from build123d import *

# Parameters (mm, degrees)
SKETCH1_R               = 8.75
SKETCH1_R_2             = 1.5
BOSS_EXTRUDE1_DEPTH     = 8.5
CUT_EXTRUDE2_DEPTH      = 3.5
CUT_EXTRUDE2_DEPTH_BACK = 3.5
CUT_EXTRUDE2_START      = -4.25
SKETCH2_R               = 9
SKETCH2_R_2             = 6
CUT_EXTRUDE5_START      = -0.75
CUT_EXTRUDE5_DEPTH      = 7
CHAMFER1_SIZE           = 0.5


with BuildPart() as part:
    # Sketch1 → Boss-Extrude1 (new body)
    with BuildSketch(Plane(origin=(0, 0, 0), x_dir=(1, 0, 0), z_dir=(0, 1, 0))):
        with Locations(Location((0, 0, 0), (0, 0, 270))):
            Circle(SKETCH1_R)
        with Locations(Location((0, 0, 0), (0, 0, 270))):
            Circle(SKETCH1_R_2, mode=Mode.SUBTRACT)
    extrude(amount=BOSS_EXTRUDE1_DEPTH)

    # Sketch2 → Cut-Extrude2 (cut, two sides: drawn at the far end of the back side and taken through both)
    with BuildSketch(Plane(origin=(0, 8.5, 0), x_dir=(1, 0, 0), z_dir=(0, 1, 0)).offset(CUT_EXTRUDE2_START - CUT_EXTRUDE2_DEPTH_BACK)):
        Circle(SKETCH2_R)
        with Locations(Location((0, 0, 0), (0, 0, 270))):
            Circle(SKETCH2_R_2, mode=Mode.SUBTRACT)
    extrude(amount=CUT_EXTRUDE2_DEPTH + CUT_EXTRUDE2_DEPTH_BACK, mode=Mode.SUBTRACT)

    # Sketch4 → Cut-Extrude5 (cut)
    with BuildSketch(Plane(origin=(0, 8.5, 0), x_dir=(1, 0, 0), z_dir=(0, 1, 0)).offset(CUT_EXTRUDE5_START)):
        with BuildLine():
            ThreePointArc((3.526710889, 4.85410242), (3.180827716, 5.087468432), (2.81956216, 5.296231606))
            Line((2.81956216, 5.296231606), (3.230259184, 4.44607034))
            Line((3.230259184, 4.44607034), (4.165722957, 4.318188538))
            ThreePointArc((4.165722957, 4.318188538), (3.855539591, 4.597261626), (3.526710889, 4.85410242))
        make_face()
        with BuildLine():
            ThreePointArc((4.854101297, 3.526712434), (4.597261012, 3.855540323), (4.318188538, 4.165722957))
            Line((4.318188538, 4.165722957), (4.44607034, 3.230259184))
            Line((4.44607034, 3.230259184), (5.296231606, 2.81956216))
            ThreePointArc((5.296231606, 2.81956216), (5.087467925, 3.180828525), (4.854101297, 3.526712434))
        make_face()
        with BuildLine():
            ThreePointArc((1.85410212, 5.706339048), (1.453033176, 5.821399711), (1.044937393, 5.908308205))
            Line((1.044937393, 5.908308205), (1.698247753, 5.226669153))
            Line((1.698247753, 5.226669153), (2.62744432, 5.394120535))
            ThreePointArc((2.62744432, 5.394120535), (2.246204515, 5.563682708), (1.85410212, 5.706339048))
        make_face()
        with BuildLine():
            ThreePointArc((0.831973127, 5.942038431), (0.416994825, 5.98549207), (-5.4e-08, 6))
            ThreePointArc((-5.4e-08, 6), (-0.416994879, 5.985492066), (-0.831973127, 5.942038431))
            Line((-0.831973127, 5.942038431), (0, 5.495645173))
            Line((0, 5.495645173), (0.831973127, 5.942038431))
        make_face()
        with BuildLine():
            Line((-1.698247753, 5.226669153), (-1.044937393, 5.908308205))
            ThreePointArc((-1.044937393, 5.908308205), (-1.453033133, 5.821399721), (-1.854102038, 5.706339075))
            ThreePointArc((-1.854102038, 5.706339075), (-2.246204475, 5.563682724), (-2.62744432, 5.394120535))
            Line((-2.62744432, 5.394120535), (-1.698247753, 5.226669153))
        make_face()
        with BuildLine():
            Line((-3.230259184, 4.44607034), (-2.81956216, 5.296231606))
            ThreePointArc((-2.81956216, 5.296231606), (-3.180828024, 5.087468239), (-3.526711477, 4.854101993))
            ThreePointArc((-3.526711477, 4.854101993), (-3.85553987, 4.597261392), (-4.165722957, 4.318188538))
            Line((-4.165722957, 4.318188538), (-3.230259184, 4.44607034))
        make_face()
        with BuildLine():
            Line((-4.44607034, 3.230259184), (-4.318188538, 4.165722957))
            ThreePointArc((-4.318188538, 4.165722957), (-4.597261623, 3.855539595), (-4.854102415, 3.526710897))
            ThreePointArc((-4.854102415, 3.526710897), (-5.087468429, 3.18082772), (-5.296231606, 2.81956216))
            Line((-5.296231606, 2.81956216), (-4.44607034, 3.230259184))
        make_face()
        with BuildLine():
            Line((-5.226669153, 1.698247753), (-5.394120535, 2.62744432))
            ThreePointArc((-5.394120535, 2.62744432), (-5.563682526, 2.246204966), (-5.706338747, 1.854103044))
            ThreePointArc((-5.706338747, 1.854103044), (-5.821399593, 1.453033647), (-5.908308205, 1.044937393))
            Line((-5.908308205, 1.044937393), (-5.226669153, 1.698247753))
        make_face()
        with BuildLine():
            ThreePointArc((5.70633865, 1.854103345), (5.563682467, 2.246205112), (5.394120535, 2.62744432))
            Line((5.394120535, 2.62744432), (5.226669153, 1.698247753))
            Line((5.226669153, 1.698247753), (5.908308205, 1.044937393))
            ThreePointArc((5.908308205, 1.044937393), (5.821399555, 1.4530338), (5.70633865, 1.854103345))
        make_face()
        with BuildLine():
            ThreePointArc((6, 0), (5.985492068, 0.416994852), (5.942038431, 0.831973127))
            Line((5.942038431, 0.831973127), (5.495645173, 0))
            Line((5.495645173, 0), (5.942038431, -0.831973127))
            ThreePointArc((5.942038431, -0.831973127), (5.985492068, -0.416994852), (6, 0))
        make_face()
        with BuildLine():
            ThreePointArc((5.706339698, -1.854100118), (5.821399966, -1.453032154), (5.908308205, -1.044937393))
            Line((5.908308205, -1.044937393), (5.226669153, -1.698247753))
            Line((5.226669153, -1.698247753), (5.394120535, -2.62744432))
            ThreePointArc((5.394120535, -2.62744432), (5.563683102, -2.246203539), (5.706339698, -1.854100118))
        make_face()
        with BuildLine():
            Line((-5.495645173, 0), (-5.942038431, 0.831973127))
            ThreePointArc((-5.942038431, 0.831973127), (-5.985492068, 0.416994852), (-6, 0))
            ThreePointArc((-6, 0), (-5.985492068, -0.416994852), (-5.942038431, -0.831973127))
            Line((-5.942038431, -0.831973127), (-5.495645173, 0))
        make_face()
        with BuildLine():
            Line((-4.44607034, -3.230259184), (-5.296231606, -2.81956216))
            ThreePointArc((-5.296231606, -2.81956216), (-5.087467714, -3.180828864), (-4.854100828, -3.526713081))
            ThreePointArc((-4.854100828, -3.526713081), (-4.597260756, -3.855540629), (-4.318188538, -4.165722957))
            Line((-4.318188538, -4.165722957), (-4.44607034, -3.230259184))
        make_face()
        with BuildLine():
            Line((-3.230259184, -4.44607034), (-4.165722957, -4.318188538))
            ThreePointArc((-4.165722957, -4.318188538), (-3.855540695, -4.5972607), (-3.52671322, -4.854100727))
            ThreePointArc((-3.52671322, -4.854100727), (-3.180828937, -5.087467668), (-2.81956216, -5.296231606))
            Line((-2.81956216, -5.296231606), (-3.230259184, -4.44607034))
        make_face()
        with BuildLine():
            Line((-1.698247753, -5.226669153), (-2.62744432, -5.394120535))
            ThreePointArc((-2.62744432, -5.394120535), (-2.246203408, -5.563683155), (-1.854099848, -5.706339786))
            ThreePointArc((-1.854099848, -5.706339786), (-1.453032017, -5.8214), (-1.044937393, -5.908308205))
            Line((-1.044937393, -5.908308205), (-1.698247753, -5.226669153))
        make_face()
        with BuildLine():
            Line((0, -5.495645173), (-0.831973127, -5.942038431))
            ThreePointArc((-0.831973127, -5.942038431), (-0.416994852, -5.985492068), (1e-09, -6))
            ThreePointArc((1e-09, -6), (0.416994853, -5.985492068), (0.831973127, -5.942038431))
            Line((0.831973127, -5.942038431), (0, -5.495645173))
        make_face()
        with BuildLine():
            ThreePointArc((1.854099793, -5.706339804), (2.246203381, -5.563683166), (2.62744432, -5.394120535))
            Line((2.62744432, -5.394120535), (1.698247753, -5.226669153))
            Line((1.698247753, -5.226669153), (1.044937393, -5.908308205))
            ThreePointArc((1.044937393, -5.908308205), (1.453031988, -5.821400007), (1.854099793, -5.706339804))
        make_face()
        with BuildLine():
            ThreePointArc((3.526713316, -4.854100657), (3.855540741, -4.597260662), (4.165722957, -4.318188538))
            Line((4.165722957, -4.318188538), (3.230259184, -4.44607034))
            Line((3.230259184, -4.44607034), (2.81956216, -5.296231606))
            ThreePointArc((2.81956216, -5.296231606), (3.180828987, -5.087467637), (3.526713316, -4.854100657))
        make_face()
        with BuildLine():
            ThreePointArc((4.854100726, -3.52671322), (5.087467668, -3.180828937), (5.296231606, -2.81956216))
            Line((5.296231606, -2.81956216), (4.44607034, -3.230259184))
            Line((4.44607034, -3.230259184), (4.318188538, -4.165722957))
            ThreePointArc((4.318188538, -4.165722957), (4.5972607, -3.855540695), (4.854100726, -3.52671322))
        make_face()
        Polygon((-5.226669153, -1.698247753), (-5.415863123, -2.748095092), (-5.996815072, -0.960108841), align=None)
    extrude(amount=-CUT_EXTRUDE5_DEPTH, mode=Mode.SUBTRACT)

    # Chamfer1
    chamfer1_edges = [part.edges().sort_by_distance(p)[0] for p in [
        (0, 0, -1.5),
        (0, 8.5, -1.5),
    ]]
    chamfer(chamfer1_edges, length=CHAMFER1_SIZE)


solid = part.part
Geometry check sheet. Reference: the model listing, model coordinates, mm. A direction names the side the tool comes from. Give positions to 0.01 mm unless a question says otherwise; leave off trailing zeros. Loops run counter-clockwise (first coordinate to the right, second up) from the corner with the lowest first, then second, coordinate; pieces in that order, holes last. Notation, with made-up numbers: (54.5, -23) -> (81.5, -23) arc R23 cw to (81.5, -11) -> close; hole circle Ø10 at (84.25, 69). An arc over 180 degrees is marked (long way). Answer in a Markdown table with one row per item. Add a question column.
1) Material ranges on probe 1 along Y at (x, z) = (5.75, 2.5); probe 2 along X at (y, z) = (4.5, 1); probe 3 along Z at (x, y) = (0.5, 3), recorded low to high. Write a range as from..to.
2) Cross-section at A-A on z = -7.5. Record the boundary of the cut face in (x, y).
3) Cross-section at B-B on x = -7.25. Record the boundary of the cut face in (y, z).
4) Set-up check for faces 1 (the face through (0.42, 4.3, 5.72)), 2 (the face through (0, 0.75, 6)), 3 (the face through (5.31, 4.3, -2.17)): record each of +Z, -Z, +X, -X, +Y, -Y from which the full face is reachable in a straight line by a thin tool's end or side.
5) Draft check along Z on faces 4 (the face through (-4.383, 4.299, -3.691)), 5 (the face through (-3.02, 4.3, 4.88)), 6 (the face through (5.716, 4.299, 0.41)). Enter one of: pulls with the +Z half, pulls with the -Z half, needs draft (parallel to the pull), parting line crosses it, or undercut.
6) Gauge pin test, flat ends, axial feed: P1, Ø5, axis at y = 5, z = 5.5, coming from the -X side; P2, Ø4, axis at x = 6.5, y = 5, coming from the +Z side. Record the tip position at first contact, or that the pin passes through.
7) Cross-section at C-C on x = 3.5. Record the boundary of the cut face in (y, z).
Outcome:
| question | item | result |
|---|---|---|
| 1 | probe 1 | y = 0..0.75, 7.75..8.5 |
| 1 | probe 2 | x = -5.92..-1.12, 1.12..5.92 |
| 1 | probe 3 | z = -5.76..-1.41, 1.41..5.76 |
| 2 | outline | (-4.51, 0) -> (4.51, 0) -> (4.51, 0.75) -> (-4.51, 0.75) -> close; (-4.51, 7.75) -> (4.51, 7.75) -> (4.51, 8.5) -> (-4.51, 8.5) -> close |
| 3 | outline | (0, -4.9) -> (0.75, -4.9) -> (0.75, 4.9) -> (0, 4.9) -> close; (7.75, -4.9) -> (8.5, -4.9) -> (8.5, 4.9) -> (7.75, 4.9) -> close |
| 4 | face 1 | +Z |
| 4 | face 2 | none |
| 4 | face 3 | +X |
| 5 | face 4 | pulls with the -Z half |
| 5 | face 5 | pulls with the +Z half |
| 5 | face 6 | undercut |
| 6 | P1 | stops at x = -4.92 |
| 6 | P2 | stops at z = 3.2 |
| 7 | outline | (0, -8.02) -> (0.75, -8.02) -> (0.75, -4.41) -> (7.75, -4.41) -> (7.75, -8.02) -> (8.5, -8.02) -> (8.5, 8.02) -> (7.75, 8.02) -> (7.75, 4.41) -> (0.75, 4.41) -> (0.75, 8.02) -> (0, 8.02) -> close |
